Build history of the part. All positions in model axes, mm. A direction names the side the tool comes from. Round coordinates to 2 decimals unless told otherwise and drop trailing zeros. Write each loop counter-clockwise with the first axis right and the second up, starting at its lowest first coordinate (ties: lowest second). Pieces come first, ordered by that corner, then holes. Notation, with made-up numbers: M 13.5,80.25 L 32.5,80.25 A11 cw 32.5,90.25 Z; hole C -38,-18.5 d9. An arc over 180 degrees is marked long. Use a Markdown table: item, result.
from build123d import *

# Parameters (mm, degrees)
SKETCH_1_R         = 22
SKETCH_1_R_2       = 12.5
EXTRUDE_1_DEPTH    = 3
EXTRUDE_2_DEPTH    = 8
HOLE_WIZARD_M3_1_D = 3.2


with BuildPart() as part:
    # ｽｹｯﾁ1 → ﾎﾞｽ - 押し出し1 (new body)
    with BuildSketch(Plane.XY):
        Circle(SKETCH_1_R)
        Circle(SKETCH_1_R_2, mode=Mode.SUBTRACT)
    extrude(amount=EXTRUDE_1_DEPTH)

    # ｽｹｯﾁ1<4> → ﾎﾞｽ - 押し出し2 (add)
    with BuildSketch(Plane.XY):
        with BuildLine():
            ThreePointArc((-20.5, 0), (-17.753520778, -10.25), (-10.25, -17.753520778))
            ThreePointArc((-10.25, -17.753520778), (-6.151923789, -16.655444566), (-7.25, -12.557368355))
            ThreePointArc((-7.25, -12.557368355), (-12.557368355, -7.25), (-14.5, 0))
            ThreePointArc((-14.5, 0), (-17.5, 3), (-20.5, 0))
        make_face()
        with BuildLine():
            ThreePointArc((10.25, 17.753520778), (0, 20.5), (-10.25, 17.753520778))
            ThreePointArc((-10.25, 17.753520778), (-11.348076211, 13.655444566), (-7.25, 12.557368355))
            ThreePointArc((-7.25, 12.557368355), (0, 14.5), (7.25, 12.557368355))
            ThreePointArc((7.25, 12.557368355), (11.348076211, 13.655444566), (10.25, 17.753520778))
        make_face()
        with BuildLine():
            ThreePointArc((10.25, -17.753520778), (17.753520778, -10.25), (20.5, 0))
            ThreePointArc((20.5, 0), (17.5, 3), (14.5, 0))
            ThreePointArc((14.5, 0), (12.557368355, -7.25), (7.25, -12.557368355))
            ThreePointArc((7.25, -12.557368355), (6.151923789, -16.655444566), (10.25, -17.753520778))
        make_face()
    extrude(amount=EXTRUDE_2_DEPTH)

    # M3 すきま穴1 (through all)
    with Locations(Plane(origin=(8.75, 15.155444566, 0), x_dir=(-1, 0, 0), z_dir=(0, 0, -1))):
        with Locations((0, 0), (-8.75, -15.155444566), (0, -30.310889132), (17.5, -30.310889132), (26.25, -15.155444566), (17.5, 0)):
            Hole(HOLE_WIZARD_M3_1_D / 2)


solid = part.part
Q1. Cut at C-C on y = 1. Give the cut face in (x, z), and give its area (3 significant figures).
Response values:
| item | result |
|---|---|
| outline | M -21.98,0 L -18.75,0 L -18.75,8 L -20.33,8 L -20.33,3 L -21.98,3 Z; M -16.25,0 L -12.46,0 L -12.46,3 L -14.67,3 L -14.67,8 L -16.25,8 Z; M 12.46,0 L 16.25,0 L 16.25,8 L 14.67,8 L 14.67,3 L 12.46,3 Z; M 18.75,0 L 21.98,0 L 21.98,3 L 20.33,3 L 20.33,8 L 18.75,8 Z |
| area | 73.7 mm2 |
Q2. Cut at D-D on x = -9. Give the cut face in (y, z) (3 decimals), and give its area (3 significant figures).
Response values:
| item | result |
|---|---|
| outline | M -20.075,0 L -16.736,0 L -16.736,8 L -18.145,8 L -18.145,3 L -20.075,3 Z; M -13.575,0 L -8.675,0 L -8.675,3 L -11.369,3 L -11.369,8 L -13.575,8 Z; M 8.675,0 L 13.575,0 L 13.575,8 L 12.166,8 L 12.166,3 L 8.675,3 Z; M 16.736,0 L 20.075,0 L 20.075,3 L 18.419,3 L 18.419,8 L 16.736,8 Z |
| area | 83.0 mm2 |
Q3. Drill centre lines: L1, parallel to X at y = 0.5, z = 7.75; L2, parallel to Y at x = 8.75, z = 4.25; L3, parallel to Y at x = -8, z = 6.75. Where is each one in solid material? Low to high.
Response values:
| item | result |
|---|---|
| L1 | x = -20.46 to -19.02, -15.98 to -14.54, 14.54 to 15.98, 19.02 to 20.46 |
| L2 | y = -18.16 to -16.76, -13.56 to -11.56, 12.16 to 13.56, 16.76 to 18.54 |
| L3 | y = -18.06 to -16.57, -13.74 to -12.09, 12.25 to 13.74, 16.57 to 18.87 |
Q4. Two-plate mould, pull along X, no slides. Class faces 4 (the cylindrical face through (11.923, 3.755, 1.479)), 5 (the cylindrical face through (-4.769, -21.477, 1.479)), 6 (the flat face through (9, -9, 0)), 7 (the cylindrical face through (7.571, -14.074, 4.056)): +X half, -X half, draft (parallel to the pull), parting line (faces both ways), or undercut.
Response values:
| item | result |
|---|---|
| face 4 | undercut |
| face 5 | parting line |
| face 6 | draft |
| face 7 | undercut |
Q5. Cut at B-B on z = 4.5. Count the separate pieces of the cut face and the enclosed holes in it, and give its area (3 significant figures).
Response values:
| item | result |
|---|---|
| separate pieces | 3 |
| enclosed holes | 6 |
| area | 366 mm2 |
Q6. Which spindle directions (+Z, -Z, +X, -X, +Y, -Y) get a long thin tool onto all of the face, cutting with end or side? Do faces 1 (the cylindrical face through (6.12, -16.6, 5.46)), 2 (the cylindrical face through (17.6, 3, 5.5)), 3 (the cylindrical face through (-17.83, -10.12, 5.46)). Say none if no direction does.
Response values:
| item | result |
|---|---|
| face 1 | +Z |
| face 2 | +Z, +Y |
| face 3 | +Z, -X, -Y |
Q7. Cut at A-A on x = 0. Give the cut face in (y, z).
Response values:
| item | result |
|---|---|
| outline | M -22,0 L -12.5,0 L -12.5,3 L -22,3 Z; M 12.5,0 L 22,0 L 22,3 L 20.5,3 L 20.5,8 L 14.5,8 L 14.5,3 L 12.5,3 Z |
Q8. Drop flat-ended pins along their axis: P1, Ø3, axis at x = 8.75, y = -15.16, coming from the -Z side (3 decimals); P2, Ø1, axis at x = 5, z = 1.5, coming from the -Y side; P3, Ø3, axis at x = -8.5, z = 3, coming from the +Y side; P4, Ø1, axis at x = -1.5, z = 1.5, coming from the +Y side. Give the stop position or say it passes through.
Response values:
| item | result |
|---|---|
| P1 | passes through |
| P2 | stops at y = -21.53 |
| P3 | stops at y = 20.86 |
| P4 | stops at y = 21.98 |
